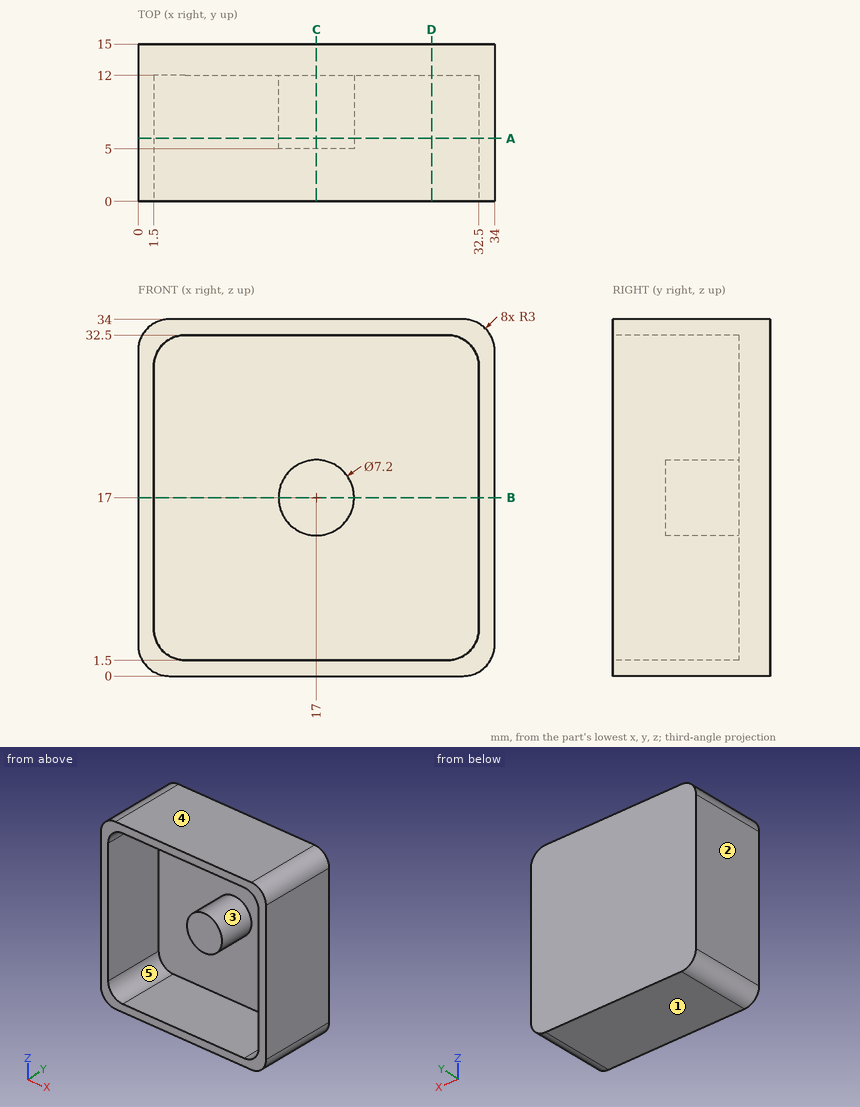
Could you check a few things on this drawing? It's one solid part, dimensions in mm from its lowest x, y, z. A direction names the side the tool comes from. Round coordinates to 2 decimals unless told otherwise and drop trailing zeros. Order: outer loops, then holes, each group sorted by start corner. A loop starts at its lowest first (then second) coordinate and runs counter-clockwise, first axis right, second up. Notation, with made-up numbers: M -26.75,55 L 7.25,55 A14 cw 7.25,59 Z; hole C -5.75,17 d8. An arc over 180 degrees is marked long. One line per question, with ' | ' between items.
1) I'm going to push a flat-ended pin straight in: pin 1 Ø2 at (x, z) = (17, 18) entering from -Y. Where does the tip first touch, or does it pass through?
Checked values:
pin 1: stops at y = 5
2) Imagine slicing it at D-D, the plane x = 28. Write out the boundary of the cut face in (y, z).
Checked values:
outline: M 0,0 L 15,0 L 15,34 L 0,34 L 0,32.5 L 12,32.5 L 12,1.5 L 0,1.5 Z
3) Imagine slicing it at B-B, the plane z = 17. Write out the boundary of the cut face in (x, y), plus the area to 3 significant figures.
Checked values:
outline: M 0,0 L 1.5,0 L 1.5,12 L 13.4,12 L 13.4,5 L 20.6,5 L 20.6,12 L 32.5,12 L 32.5,0 L 34,0 L 34,15 L 0,15 Z | area: 188 mm²
4) Imagine slicing it at A-A, the plane y = 6. Write out the boundary of the cut face in (x, z).
Checked values:
outline: M 0,3 A3 ccw 3,0 L 31,0 A3 ccw 34,3 L 34,31 A3 ccw 31,34 L 3,34 A3 ccw 0,31 Z; C 17,17 d7.2; hole M 1.5,4.5 A3 ccw 4.5,1.5 L 29.5,1.5 A3 ccw 32.5,4.5 L 32.5,29.5 A3 ccw 29.5,32.5 L 4.5,32.5 A3 ccw 1.5,29.5 Z
5) I need wall thicknesses on line 1 (Z direction, x = 18, y = 9.75); line 2 (Z direction, x = 20.5, y = 3.5). Which ranges of each line are inside material? Lowest first, please.
Checked values:
line 1: z = 0 to 1.5, 13.54 to 20.46, 32.5 to 34 | line 2: z = 0 to 1.5, 32.5 to 34
6) We'd pull the mould along X, two halves only. Please class the marked faces 1, 2 and 3: released by +X, released by -X, zero draft, split by the parting line, or undercut.
Checked values:
face 1: zero draft | face 2: released by -X | face 3: undercut
7) Imagine slicing it at C-C, the plane x = 17. Write out the boundary of the cut face in (y, z).
Checked values:
outline: M 0,0 L 15,0 L 15,34 L 0,34 L 0,32.5 L 12,32.5 L 12,20.6 L 5,20.6 L 5,13.4 L 12,13.4 L 12,1.5 L 0,1.5 Z
8) On a 3-axis mill with a long thin cutter (end or side, diameter ignored), from which of +Z, -Z, +X, -X, +Y, -Y can I reach the whole of each face in a straight line? I mean the marked faces 4 and 5. Say none if no direction works.
Checked values:
face 4: +Z, +X, -X, +Y, -Y | face 5: -Y
